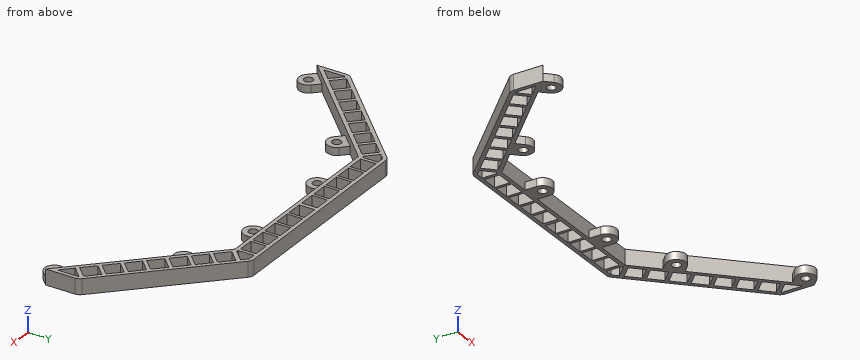
from build123d import *

# Parameters (mm, degrees)
SKETCH3_R                = 1.15
BOSS_EXTRUDE1_DEPTH      = 2
CUT_EXTRUDE4_DEPTH       = 2
FILLET1_R                = 2
CUT_EXTRUDE1_DEPTH       = 83.231380871
CUT_EXTRUDE2_DEPTH       = 83.158383626
LPATTERN1_COUNT          = 7
LPATTERN1_PITCH          = 5
SKETCH7_W                = 4.2
SKETCH7_H                = 4
CUT_EXTRUDE3_DEPTH       = 83.158383626
LPATTERN2_COUNT          = 5
LPATTERN2_PITCH          = 4.9
MIRROR1_COPY_1_DEPTH     = 83.158383626
MIRROR1_COPY_2_DEPTH     = 83.158383626
MIRROR1_COPY_3_DEPTH     = 83.158383626
MIRROR1_COPY_4_DEPTH     = 83.158383626
MIRROR1_COPY_5_DEPTH     = 83.158383626
MIRROR1_COPY_6_DEPTH     = 83.158383626
MIRROR1_COPY_7_SKETCH_W  = 4.2
MIRROR1_COPY_7_SKETCH_H  = 4
MIRROR1_COPY_7_DEPTH     = 83.158383626
MIRROR1_COPY_8_SKETCH_W  = 4.2
MIRROR1_COPY_8_SKETCH_H  = 4
MIRROR1_COPY_8_DEPTH     = 83.158383626
MIRROR1_COPY_9_SKETCH_W  = 4.2
MIRROR1_COPY_9_SKETCH_H  = 4
MIRROR1_COPY_9_DEPTH     = 83.158383626
MIRROR1_COPY_10_SKETCH_W = 4.2
MIRROR1_COPY_10_SKETCH_H = 4
MIRROR1_COPY_10_DEPTH    = 83.158383626
FILLET1_OF_MIRROR1_R     = 2


with BuildPart() as part:
    # Sketch3 → Boss-Extrude1 (new, symmetric)
    with BuildSketch(Plane.XY):
        with BuildLine():
            Line((-55, 25), (-53.25, 23.25))
            ThreePointArc((-53.25, 23.25), (-49.75, 23.25), (-49.75, 26.75))
            Line((-49.75, 26.75), (-51.5, 28.5))
            Line((-51.5, 28.5), (-34.517766953, 45.482233047))
            Line((-34.517766953, 45.482233047), (-32.767766953, 43.732233047))
            ThreePointArc((-32.767766953, 43.732233047), (-29.232233047, 43.732233047), (-29.232233047, 47.267766953))
            Line((-29.232233047, 47.267766953), (-30.982233047, 49.017766953))
            Line((-30.982233047, 49.017766953), (-25, 55))
            Line((-25, 55), (-15.5, 55))
            Line((-15.5, 55), (-15.5, 52))
            ThreePointArc((-15.5, 52), (-13, 49.5), (-10.5, 52))
            Line((-10.5, 52), (-10.5, 55))
            Line((-10.5, 55), (0, 55))
            Line((0, 55), (0, 61))
            Line((0, 61), (-27.485281374, 61))
            Line((-27.485281374, 61), (-55, 33.485281374))
            Line((-55, 33.485281374), (-55, 25))
        make_face()
        with Locations((-13, 52)):
            Circle(SKETCH3_R, mode=Mode.SUBTRACT)
        with Locations((-31, 45.5)):
            Circle(SKETCH3_R, mode=Mode.SUBTRACT)
        with Locations((-51.5, 25)):
            Circle(SKETCH3_R, mode=Mode.SUBTRACT)
    boss_extrude1 = extrude(amount=BOSS_EXTRUDE1_DEPTH, both=True)

    # Sketch8 → Cut-Extrude4 (cut)
    with BuildSketch(Plane.XY.offset(2)):
        with BuildLine():
            Line((-55, 25), (-51.5, 28.5))
            Line((-51.5, 28.5), (-49.75, 26.75))
            ThreePointArc((-49.75, 26.75), (-49.75, 23.25), (-53.25, 23.25))
            Line((-53.25, 23.25), (-55, 25))
        make_face()
        with BuildLine():
            Line((-34.517766953, 45.482233047), (-30.982233047, 49.017766953))
            Line((-30.982233047, 49.017766953), (-29.232233047, 47.267766953))
            ThreePointArc((-29.232233047, 47.267766953), (-29.232233047, 43.732233047), (-32.767766953, 43.732233047))
            Line((-32.767766953, 43.732233047), (-34.517766953, 45.482233047))
        make_face()
        with BuildLine():
            Line((-15.5, 55), (-10.5, 55))
            Line((-10.5, 55), (-10.5, 52))
            ThreePointArc((-10.5, 52), (-13, 49.5), (-15.5, 52))
            Line((-15.5, 52), (-15.5, 55))
        make_face()
    cut_extrude4 = extrude(amount=-CUT_EXTRUDE4_DEPTH, mode=Mode.SUBTRACT)

    # Fillet1
    fillet1_edges = [part.edges().sort_by_distance(p)[0] for p in [
        (-55, 33.485281374, 0),
        (-27.485281374, 61, 0),
    ]]
    fillet(fillet1_edges, radius=FILLET1_R)

    # Sketch5 → Cut-Extrude1 (cut, through all)
    with BuildSketch(Plane.XY.offset(2)):
        Polygon((-28.428256226, 58.642811585), (-27.071067812, 60), (-25.151713549, 60), (-25.151713549, 56.019550391), (-25.613653315, 55.828208674), align=None)
        Polygon((-54, 33.071067812), (-54, 27.414213562), (-51.171572875, 30.242640687), align=None)
    cut_extrude1 = extrude(amount=-CUT_EXTRUDE1_DEPTH, mode=Mode.SUBTRACT)

    # Sketch6 → Cut-Extrude2 (cut, symmetric)
    with BuildSketch(Plane.XY):
        Polygon((-53.292893219, 33.778174593), (-50.393755416, 36.677312396), (-47.565328291, 33.848885271), (-50.464466094, 30.949747468), align=None)
    cut_extrude2 = extrude(amount=CUT_EXTRUDE2_DEPTH, both=True, mode=Mode.SUBTRACT)

    # LPattern1: Cut-Extrude2 ×7
    with Locations(*[Vector(0.7071067811865472, 0.7071067811865478, 0) * (i * LPATTERN1_PITCH) for i in range(1, LPATTERN1_COUNT)]):
        add(cut_extrude2, mode=Mode.SUBTRACT)

    # Sketch7 → Cut-Extrude3 (cut, symmetric)
    with BuildSketch(Plane.XY):
        with Locations((-2.6, 58)):
            Rectangle(SKETCH7_W, SKETCH7_H)
    cut_extrude3 = extrude(amount=CUT_EXTRUDE3_DEPTH, both=True, mode=Mode.SUBTRACT)

    # LPattern2: Cut-Extrude3 ×5
    with Locations(*[(-i * LPATTERN2_PITCH, 0, 0) for i in range(1, LPATTERN2_COUNT)]):
        add(cut_extrude3, mode=Mode.SUBTRACT)

    # Mirror1: Boss-Extrude1, Cut-Extrude4, Cut-Extrude1, Cut-Extrude2, Cut-Extrude3 across plane
    add(boss_extrude1.mirror(Plane(origin=(0, 55, 2), x_dir=(0, 0, 1), z_dir=(-1, 0, 0))))
    add(cut_extrude4.mirror(Plane(origin=(0, 55, 2), x_dir=(0, 0, 1), z_dir=(-1, 0, 0))), mode=Mode.SUBTRACT)
    add(cut_extrude1.mirror(Plane(origin=(0, 55, 2), x_dir=(0, 0, 1), z_dir=(-1, 0, 0))), mode=Mode.SUBTRACT)
    add(cut_extrude2.mirror(Plane(origin=(0, 55, 2), x_dir=(0, 0, 1), z_dir=(-1, 0, 0))), mode=Mode.SUBTRACT)
    add(cut_extrude3.mirror(Plane(origin=(0, 55, 2), x_dir=(0, 0, 1), z_dir=(-1, 0, 0))), mode=Mode.SUBTRACT)

    # Mirror1 copy 1 sketch → Mirror1 copy 1 (cut, symmetric)
    with BuildSketch(Plane(origin=(-3.535533906, 3.535533906, 0), x_dir=(-1, 0, 0), z_dir=(0, 0, 1))):
        Polygon((-53.292893219, -33.778174593), (-50.393755416, -36.677312396), (-47.565328291, -33.848885271), (-50.464466094, -30.949747468), align=None)
    extrude(amount=MIRROR1_COPY_1_DEPTH, both=True, mode=Mode.SUBTRACT)

    # Mirror1 copy 2 sketch → Mirror1 copy 2 (cut, symmetric)
    with BuildSketch(Plane(origin=(-7.071067812, 7.071067812, 0), x_dir=(-1, 0, 0), z_dir=(0, 0, 1))):
        Polygon((-53.292893219, -33.778174593), (-50.393755416, -36.677312396), (-47.565328291, -33.848885271), (-50.464466094, -30.949747468), align=None)
    extrude(amount=MIRROR1_COPY_2_DEPTH, both=True, mode=Mode.SUBTRACT)

    # Mirror1 copy 3 sketch → Mirror1 copy 3 (cut, symmetric)
    with BuildSketch(Plane(origin=(-10.606601718, 10.606601718, 0), x_dir=(-1, 0, 0), z_dir=(0, 0, 1))):
        Polygon((-53.292893219, -33.778174593), (-50.393755416, -36.677312396), (-47.565328291, -33.848885271), (-50.464466094, -30.949747468), align=None)
    extrude(amount=MIRROR1_COPY_3_DEPTH, both=True, mode=Mode.SUBTRACT)

    # Mirror1 copy 4 sketch → Mirror1 copy 4 (cut, symmetric)
    with BuildSketch(Plane(origin=(-14.142135624, 14.142135624, 0), x_dir=(-1, 0, 0), z_dir=(0, 0, 1))):
        Polygon((-53.292893219, -33.778174593), (-50.393755416, -36.677312396), (-47.565328291, -33.848885271), (-50.464466094, -30.949747468), align=None)
    extrude(amount=MIRROR1_COPY_4_DEPTH, both=True, mode=Mode.SUBTRACT)

    # Mirror1 copy 5 sketch → Mirror1 copy 5 (cut, symmetric)
    with BuildSketch(Plane(origin=(-17.67766953, 17.67766953, 0), x_dir=(-1, 0, 0), z_dir=(0, 0, 1))):
        Polygon((-53.292893219, -33.778174593), (-50.393755416, -36.677312396), (-47.565328291, -33.848885271), (-50.464466094, -30.949747468), align=None)
    extrude(amount=MIRROR1_COPY_5_DEPTH, both=True, mode=Mode.SUBTRACT)

    # Mirror1 copy 6 sketch → Mirror1 copy 6 (cut, symmetric)
    with BuildSketch(Plane(origin=(-21.213203436, 21.213203436, 0), x_dir=(-1, 0, 0), z_dir=(0, 0, 1))):
        Polygon((-53.292893219, -33.778174593), (-50.393755416, -36.677312396), (-47.565328291, -33.848885271), (-50.464466094, -30.949747468), align=None)
    extrude(amount=MIRROR1_COPY_6_DEPTH, both=True, mode=Mode.SUBTRACT)

    # Mirror1 copy 7 sketch → Mirror1 copy 7 (cut, symmetric)
    with BuildSketch(Plane(origin=(4.9, 0, 0), x_dir=(-1, 0, 0), z_dir=(0, 0, 1))):
        with Locations((-2.6, -58)):
            Rectangle(MIRROR1_COPY_7_SKETCH_W, MIRROR1_COPY_7_SKETCH_H)
    extrude(amount=MIRROR1_COPY_7_DEPTH, both=True, mode=Mode.SUBTRACT)

    # Mirror1 copy 8 sketch → Mirror1 copy 8 (cut, symmetric)
    with BuildSketch(Plane(origin=(9.8, 0, 0), x_dir=(-1, 0, 0), z_dir=(0, 0, 1))):
        with Locations((-2.6, -58)):
            Rectangle(MIRROR1_COPY_8_SKETCH_W, MIRROR1_COPY_8_SKETCH_H)
    extrude(amount=MIRROR1_COPY_8_DEPTH, both=True, mode=Mode.SUBTRACT)

    # Mirror1 copy 9 sketch → Mirror1 copy 9 (cut, symmetric)
    with BuildSketch(Plane(origin=(14.7, 0, 0), x_dir=(-1, 0, 0), z_dir=(0, 0, 1))):
        with Locations((-2.6, -58)):
            Rectangle(MIRROR1_COPY_9_SKETCH_W, MIRROR1_COPY_9_SKETCH_H)
    extrude(amount=MIRROR1_COPY_9_DEPTH, both=True, mode=Mode.SUBTRACT)

    # Mirror1 copy 10 sketch → Mirror1 copy 10 (cut, symmetric)
    with BuildSketch(Plane(origin=(19.6, 0, 0), x_dir=(-1, 0, 0), z_dir=(0, 0, 1))):
        with Locations((-2.6, -58)):
            Rectangle(MIRROR1_COPY_10_SKETCH_W, MIRROR1_COPY_10_SKETCH_H)
    extrude(amount=MIRROR1_COPY_10_DEPTH, both=True, mode=Mode.SUBTRACT)

    # Fillet1 of Mirror1
    fillet1_of_mirror1_edges = [part.edges().sort_by_distance(p)[0] for p in [
        (55, 33.485281374, 0),
        (27.485281374, 61, 0),
    ]]
    fillet(fillet1_of_mirror1_edges, radius=FILLET1_OF_MIRROR1_R)


solid = part.part
Build history of the part. All positions in model axes, mm. Coordinates: 2 decimals unless noted, no trailing zeros. Order: outer loops, then holes, each group sorted by start corner. A loop starts at its lowest first (then second) coordinate and runs counter-clockwise, first axis right, second up. Notation, with made-up numbers: (29.25, -7) - (62.25, -7) arc R18 cw to (62.25, 22) - close; hole circle Ø3 at (70.25, 75.5). An arc over 180 degrees is marked (long way). Write each question's results on one line, items separated by ' | '. Start each with the question number.
Item 1: Band-saw the part on C-C on z = -1. State how many separate pieces and enclosed holes the cut face has, and give its area (3 significant figures).
Item 2: Band-saw the part on B-B on x = -13. Write the cut outline in (y, z), and give its area (3 significant figures).
Item 3: Band-saw the part on A-A on x = 23. Write the cut outline in (y, z), and give its area (3 significant figures).
Item 4: Flat gauge pins, fed straight in: pin 1 (12 mm diameter, centred on x = -16, y = 42.5, fed in from +Z); pin 2 (2 mm diameter, centred on y = 58.5, z = 0.5, fed in from +X); pin 3 (2 mm diameter, centred on y = 57.5, z = 0, fed in from +X); pin 4 (2 mm diameter, centred on y = 57, z = 0.5, fed in from +X). Where does each tip first touch, or does it go through?
Item 5: Wall check: probe 1 along Y at (x, z) = (-13, -1); probe 2 along X at (y, z) = (31.5, -1.2); probe 3 along X at (y, z) = (29.5, 0.95). Give the ranges that are in metal, low to high. Write a range as [from, to].
Numbers:
1) separate pieces: 1 | enclosed holes: 34 | area: 484 mm^2
2) outline: (49.5, -2) - (50.85, -2) - (50.85, 0) - (49.5, 0) - close; (53.15, -2) - (56, -2) - (56, 2) - (55, 2) - (55, 0) - (53.15, 0) - close; (60, -2) - (61, -2) - (61, 2) - (60, 2) - close | area: 14.4 mm^2
3) outline: (55, -2) - (56, -2) - (56, 2) - (55, 2) - close; (60, -2) - (61, -2) - (61, 2) - (60, 2) - close | area: 8.00 mm^2
4) pin 1: through | pin 2: x = 30.99 | pin 3: x = 31.99 | pin 4: x = 32.49
5) probe 1: [49.5, 50.85], [53.15, 56], [60, 61] | probe 2: [-55, -54], [-52.43, -51.01], [-49.91, -48.5], [48.5, 49.91], [51.01, 52.43], [54, 55] | probe 3: [-55, -54], [-51.91, -50.5], [50.5, 51.91], [54, 55]
